from build123d import *

# Parameters (mm, degrees)
SKETCH1_W           = 36.1
SKETCH1_H           = 36.1
SKETCH1_R           = 1.025
BOSS_EXTRUDE1_DEPTH = 3
SKETCH1_3_W         = 36.1
SKETCH1_3_H         = 36.1
SKETCH1_3_W_2       = 32.1
SKETCH1_3_H_2       = 32.1
BOSS_EXTRUDE2_DEPTH = 8.15
SKETCH2_W           = 17
SKETCH2_H           = 3.65
CUT_EXTRUDE1_DEPTH  = 6
CUT_EXTRUDE2_DEPTH  = 1
SKETCH6_W           = 3
SKETCH6_H           = 10
BOSS_EXTRUDE3_DEPTH = 10.2
FILLET1_R           = 5
SKETCH7_R           = 1.5
CUT_EXTRUDE3_DEPTH  = 10
CHAMFER1_SIZE2      = 1
CHAMFER1_SIZE       = 1.85


with BuildPart() as part:
    # Sketch1 → Boss-Extrude1 (new body)
    with BuildSketch(Plane(origin=(0, 0, 0), x_dir=(1, 0, 0), z_dir=(0, 1, 0))):
        Rectangle(SKETCH1_W, SKETCH1_H)
        with Locations(Location((-14, 14, 0), (0, 0, 270))):
            Circle(SKETCH1_R, mode=Mode.SUBTRACT)
        with Locations(Location((14, 14, 0), (0, 0, 270))):
            Circle(SKETCH1_R, mode=Mode.SUBTRACT)
        with Locations(Location((14, -14, 0), (0, 0, 270))):
            Circle(SKETCH1_R, mode=Mode.SUBTRACT)
        with Locations(Location((-14, -14, 0), (0, 0, 270))):
            Circle(SKETCH1_R, mode=Mode.SUBTRACT)
        with BuildLine():
            Line((-8.64, 2.4), (-8.64, 8.64))
            Line((-8.64, 8.64), (8.64, 8.64))
            Line((8.64, 8.64), (8.64, 2.4))
            Line((8.64, 2.4), (10, 2.4))
            ThreePointArc((10, 2.4), (12.4, 0), (10, -2.4))
            Line((10, -2.4), (8.64, -2.4))
            Line((8.64, -2.4), (8.64, -8.64))
            Line((8.64, -8.64), (-8.64, -8.64))
            Line((-8.64, -8.64), (-8.64, -2.4))
            Line((-8.64, -2.4), (-10, -2.4))
            ThreePointArc((-10, -2.4), (-12.4, 0), (-10, 2.4))
            Line((-10, 2.4), (-8.64, 2.4))
        make_face(mode=Mode.SUBTRACT)
    extrude(amount=BOSS_EXTRUDE1_DEPTH)

    # Sketch1<3> → Boss-Extrude2 (add)
    with BuildSketch(Plane(origin=(0, 0, 0), x_dir=(1, 0, 0), z_dir=(0, 1, 0))):
        Rectangle(SKETCH1_3_W, SKETCH1_3_H)
        Rectangle(SKETCH1_3_W_2, SKETCH1_3_H_2, mode=Mode.SUBTRACT)
    extrude(amount=BOSS_EXTRUDE2_DEPTH)

    # Sketch2 → Cut-Extrude1 (cut)
    with BuildSketch(Plane(origin=(0, 0, -18.05), x_dir=(-1, 0, 0), z_dir=(0, 0, -1))):
        with Locations((0, 6.325)):
            Rectangle(SKETCH2_W, SKETCH2_H)
    extrude(amount=-CUT_EXTRUDE1_DEPTH, mode=Mode.SUBTRACT)

    # Sketch4 → Cut-Extrude2 (cut)
    with BuildSketch(Plane(origin=(0, 8.15, 0), x_dir=(1, 0, 0), z_dir=(0, 1, 0))):
        Polygon((17.05, -17.05), (-17.05, -17.05), (-17.05, 17.05), (-8.5, 17.05), (-8.5, 16.05), (-16.05, 16.05), (-16.05, -16.05), (16.05, -16.05), (16.05, 16.05), (8.5, 16.05), (8.5, 17.05), (17.05, 17.05), align=None)
    extrude(amount=-CUT_EXTRUDE2_DEPTH, mode=Mode.SUBTRACT)

    # Sketch6 → Boss-Extrude3 (add)
    with BuildSketch(Plane.XY.offset(18.05)):
        with Locations((1.5, 5)):
            Rectangle(SKETCH6_W, SKETCH6_H)
    extrude(amount=BOSS_EXTRUDE3_DEPTH)

    # Fillet1
    fillet1_edges = [part.edges().sort_by_distance(p)[0] for p in [
        (1.5, 0, 28.25),
        (1.5, 10, 28.25),
    ]]
    fillet(fillet1_edges, radius=FILLET1_R - 0.0001)  # a hair under: the kernel refuses the full size

    # Sketch7 → Cut-Extrude3 (cut)
    with BuildSketch(Plane(origin=(3, 0, 0), x_dir=(0, 0, -1), z_dir=(1, 0, 0))):
        with Locations(Location((-23.25, 5, 0), (0, 0, 90))):
            Circle(SKETCH7_R)
    extrude(amount=-CUT_EXTRUDE3_DEPTH, mode=Mode.SUBTRACT)

    # Chamfer1
    chamfer1_edges = [part.edges().sort_by_distance(p)[0] for p in [
        (1.5, 8.15, 18.05),
    ]]
    chamfer1_side = [part.faces().sort_by_distance(p)[0] for p in [
        (1.5, 8.17, 18.05),
    ]]
    chamfer(chamfer1_edges, length=CHAMFER1_SIZE - 0.0001, length2=CHAMFER1_SIZE2 - 0.0001, reference=chamfer1_side[0])  # a hair under: the kernel refuses the full size


solid = part.part
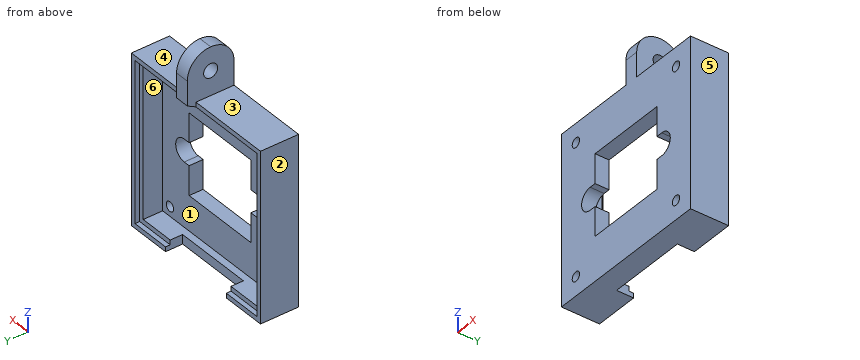
Geometry: final body of the model. Coordinates: model frame, mm. Face numbers are marked on the shaded views. A direction names the side the tool comes from. Round coordinates to 2 decimals unless told otherwise and drop trailing zeros. Loops run counter-clockwise (first coordinate to the right, second up) from the corner with the lowest first, then second, coordinate; pieces in that order, holes last.
Q1. Section B-B on x = 14. Return loops of the section in (y, z) (3 decimals).
Q2. Section C-C on z = -4. Return loops of the section in (x, y), plus the area to 3 significant figures.
Q3. Pin query (flat end, axial travel): P1, Ø0.5, axis at x = 11.5, y = 7.5, coming from the +Z side; P2, Ø12, axis at x = 14, z = 13.5, coming from the +Y side; P3, Ø8, axis at x = 1.5, z = -13, coming from the +Y side; P4, Ø1.6, axis at x = 14, z = 14, coming from the -Y side. Return the tip coordinate at first contact, or that it passes through.
Q4. Pull-direction query (X, two-part tool) for the marked faces 1, 2 and 3; classes: released by +X, released by -X, zero draft, split by the parting line, or undercut.
Q5. Material intervals for L1, parallel to X at y = 2, z = 14 (3 decimals); L2, parallel to Z at x = 8, y = 1.5; L3, parallel to X at y = 7, z = 13.5, sorted ascending.
Q6. Access query for the marked faces 4, 5 and 6. Directions: +Z, -Z, +X, -X, +Y, -Y. A direction counts if a zero-diameter tool reaches every point of the face in a straight line with its end or side. Return the directions, or none.
Q7. Section D-D on x = -0.5. Return loops of the section in (y, z), plus the area to 3 significant figures.
Q8. Section A-A on z = -14. Return loops of the section in (x, y) (3 decimals).
Evaluation:
1. outline: (0, -18.05) - (8.15, -18.05) - (8.15, -17.05) - (7.15, -17.05) - (7.15, -16.05) - (3, -16.05) - (3, -15.025) - (0, -15.025) - close; (0, -12.975) - (3, -12.975) - (3, 12.975) - (0, 12.975) - close; (0, 15.025) - (3, 15.025) - (3, 16.05) - (7.15, 16.05) - (7.15, 17.05) - (8.15, 17.05) - (8.15, 18.05) - (0, 18.05) - close
2. outline: (-18.05, 0) - (-8.64, 0) - (-8.64, 3) - (-16.05, 3) - (-16.05, 7.15) - (-17.05, 7.15) - (-17.05, 8.15) - (-18.05, 8.15) - close; (8.64, 0) - (18.05, 0) - (18.05, 8.15) - (17.05, 8.15) - (17.05, 7.15) - (16.05, 7.15) - (16.05, 3) - (8.64, 3) - close
2. area: 75.1 mm2
3. P1: stops at z = 18.05
3. P2: stops at y = 8.15
3. P3: stops at y = 4.5
3. P4: passes through
4. face 1: undercut
4. face 2: released by -X
4. face 3: zero draft
5. L1: x = -18.05 to -15.025, -12.975 to 12.975, 15.025 to 18.05
5. L2: z = -18.05 to -8.64, 8.64 to 18.05
5. L3: x = -18.05 to -16.05, 16.05 to 18.05
6. face 4: +Z, +X, +Y, -Y
6. face 5: +Z, -Z, +X, +Y, -Y
6. face 6: +Y
7. outline: (0, -18.05) - (4.5, -18.05) - (4.5, -16.05) - (3, -16.05) - (3, -8.64) - (0, -8.64) - close; (0, 8.64) - (3, 8.64) - (3, 16.05) - (7.15, 16.05) - (7.15, 17.05) - (8.15, 17.05) - (8.15, 18.05) - (0, 18.05) - close
7. area: 68.8 mm2
8. outline: (-18.05, 0) - (-15.025, 0) - (-15.025, 3) - (-16.05, 3) - (-16.05, 7.15) - (-17.05, 7.15) - (-17.05, 8.15) - (-18.05, 8.15) - close; (-12.975, 0) - (12.975, 0) - (12.975, 3) - (-12.975, 3) - close; (15.025, 0) - (18.05, 0) - (18.05, 8.15) - (17.05, 8.15) - (17.05, 7.15) - (16.05, 7.15) - (16.05, 3) - (15.025, 3) - close
